Source: CAD feature listing. Evaluate the final solid. Frame: model axes, mm. A direction names the side the tool comes from. Give positions to 0.01 mm unless a question says otherwise; leave off trailing zeros. Write each loop counter-clockwise with the first axis right and the second up, starting at its lowest first coordinate (ties: lowest second). Pieces come first, ordered by that corner, then holes. Notation, with made-up numbers: (57, 35.5) -> (93, 35.5) arc R20 ccw to (93, 42.5) -> close; hole circle Ø1 at (24.25, 51.5). An arc over 180 degrees is marked (long way). Answer as a JSON object with one key per item and string values. Group by question number.
Item 1: Section query D-D on z = 3.75. Return the cut outline in (x, y), plus the area to 3 significant figures.
Item 2: Section query B-B on z = 18.25. Return the cut outline in (x, y), plus the area to 3 significant figures.
Item 3: Access query for faces 1 (the face through (8, 0, 2)), 2 (the face through (1.568, -4.748, 3.774)), 3 (the face through (7.654, -3.143, 7.395)), 4 (the face through (2.285, 3.584, 17.712)). Directions: +Z, -Z, +X, -X, +Y, -Y. A direction counts if a zero-diameter tool reaches every point of the face in a straight line with its end or side. Return the directions, or none.
Item 4: Pull-direction query (Y, two-part tool) for faces 5 (the face through (10.492, 3.304, 3.451)), 6 (the face through (-4, -3, 4)), 7 (the face through (-3, -2, 0)), 8 (the face through (-6.73, 4.42, 2.04)); classes: pulls with the +Y half, pulls with the -Y half, needs draft (parallel to the pull), parting line crosses it, or undercut.
Item 5: Section query C-C on x = -1.5. Return the cut outline in (y, z).
Item 6: First-contact query: pin 1 Ø3 at (y, z) = (-6, 5.5) entering from -X; pin 2 Ø6 at (y, z) = (2, 14) entering from -X; pin 3 Ø4 at (y, z) = (0, 4.5) entering from +X; pin 4 Ø1.5 at (x, z) = (-4.5, 18.5) entering from -Y. Flat tips, straight axial feed; report the tip coordinate or a pass-through.
Item 7: Ray query, probe 1 along X at (y, z) = (-3, 7.5); probe 2 along Y at (x, z) = (0, 6.25); probe 3 along Y at (x, z) = (0, 10.75). Return the intervals inside material, ascending. Write a range as from..to.
Item 8: Section query A-A on y = 0. Return the cut outline in (x, z).
from build123d import *

# Parameters (mm, degrees)
F0_R      = 11
F1_DEPTH  = 7
F2_R      = 9.5
F3_DEPTH  = 8
F4_R      = 4.25
F5_DEPTH  = 5.5
F6_R      = 3.25
F7_DEPTH  = 20.501
F10_R     = 1.75
F19_DEPTH = 6
F12_R     = 1.75
F20_DEPTH = 6
F14_R     = 1.75
F21_DEPTH = 6
F16_R     = 1.75
F22_DEPTH = 6
F18_R     = 1.75
F23_DEPTH = 6
F24_R     = 2
F25_DEPTH = 25


with BuildPart() as f1:
    # F0 (on Top) → F1 (new body)
    with BuildSketch(Plane.XY):
        Circle(F0_R)
    extrude(amount=F1_DEPTH)

    # F2 (on face) → F3 (join)
    with BuildSketch(Plane.XY.offset(7)):
        Circle(F2_R)
    extrude(amount=F3_DEPTH)

    # F4 (on face) → F5 (join)
    with BuildSketch(Plane.XY.offset(15)):
        Circle(F4_R)
    extrude(amount=F5_DEPTH)

    # F6 (on face) → F7 (cut, through all)
    with BuildSketch(Plane.XY.offset(20.5)):
        Circle(F6_R)
    extrude(amount=-F7_DEPTH, mode=Mode.SUBTRACT)

    # F10 (on line) → F19 (cut)
    with BuildSketch(Plane.YZ.offset(11)):
        with Locations((0, 3.75)):
            Circle(F10_R)
    extrude(amount=-F19_DEPTH, mode=Mode.SUBTRACT)

    # F12 (on line) → F20 (cut)
    with BuildSketch(Plane(origin=(3.3991869381, -10.4616216792, 0), x_dir=(-0.9510565163, -0.3090169944, 0), z_dir=(-0.3090169944, 0.9510565163, 0))):
        with Locations((0, 3.75)):
            Circle(F12_R)
    extrude(amount=F20_DEPTH, mode=Mode.SUBTRACT)

    # F14 (on face) → F21 (cut)
    with BuildSketch(Plane(origin=(-8.8991869381, -6.4656377752, 0), x_dir=(-0.5877852523, 0.8090169944, 0), z_dir=(0.8090169944, 0.5877852523, 0))):
        with Locations((0, 3.75)):
            Circle(F14_R)
    extrude(amount=F21_DEPTH, mode=Mode.SUBTRACT)

    # F16 (on face) → F22 (cut)
    with BuildSketch(Plane(origin=(-8.8991869381, 6.4656377752, 0), x_dir=(0.5877852523, 0.8090169944, 0), z_dir=(0.8090169944, -0.5877852523, 0))):
        with Locations((0, 3.75)):
            Circle(F16_R)
    extrude(amount=F22_DEPTH, mode=Mode.SUBTRACT)

    # F18 (on line) → F23 (cut)
    with BuildSketch(Plane(origin=(3.3991869381, 10.4616216792, 0), x_dir=(-0.9510565163, 0.3090169944, 0), z_dir=(0.3090169944, 0.9510565163, 0))):
        with Locations((0, 3.75)):
            Circle(F18_R)
    extrude(amount=-F23_DEPTH, mode=Mode.SUBTRACT)

    # F24 (on face) → F25 (cut)
    with BuildSketch(Plane(origin=(0, 0, 0), x_dir=(1, 0, 0), z_dir=(0, 0, -1))):
        with Locations((5.8068181818, 3.9090743921)):
            Circle(F24_R)
    extrude(amount=-F25_DEPTH, mode=Mode.SUBTRACT)


solid = f1.part
Worked answers:
{
 "1": {"outline": "(-9.81, -4.97) -> (-5.07, -1.52) -> (-3.02, -4.35) -> (-7.76, -7.8) arc R11 ccw to (1.69, -10.87) -> (-0.12, -5.3) -> (3.21, -4.21) -> (5.02, -9.79) arc R11 ccw to (10.86, -1.75) -> (5, -1.75) -> (5, 1.75) -> (10.86, 1.75) arc R11 ccw to (5.02, 9.79) -> (3.21, 4.21) -> (-0.12, 5.3) -> (1.69, 10.87) arc R11 ccw to (-7.76, 7.8) -> (-3.02, 4.35) -> (-5.07, 1.52) -> (-9.81, 4.97) arc R11 ccw to start; hole circle Ø6.5 at (0, 0); hole circle Ø4 at (5.81, -3.91)", "area": "230 mm^2"},
 "2": {"outline": "circle Ø8.5 at (0, 0); hole circle Ø6.5 at (0, 0)", "area": "23.6 mm^2"},
 "3": {"face 1": "+X", "face 2": "none", "face 3": "+Z, -Z", "face 4": "+Z"},
 "4": {"face 5": "parting line crosses it", "face 6": "undercut", "face 7": "needs draft", "face 8": "undercut"},
 "5": {"outline": "(-10.9, 0) -> (-2.88, 0) -> (-2.88, 20.5) -> (-3.98, 20.5) -> (-3.98, 15) -> (-9.38, 15) -> (-9.38, 7) -> (-10.9, 7) -> close; (2.88, 0) -> (10.9, 0) -> (10.9, 7) -> (9.38, 7) -> (9.38, 15) -> (3.98, 15) -> (3.98, 20.5) -> (2.88, 20.5) -> close"},
 "6": {"pin 1": "x = -10.04", "pin 2": "x = -9.5", "pin 3": "x = 11", "pin 4": "y = -2"},
 "7": {"probe 1": "-9.01..-1.25, 1.25..4.03, 7.59..9.01", "probe 2": "-11..-3.25, 3.25..11", "probe 3": "-9.5..-3.25, 3.25..9.5"},
 "8": {"outline": "(-11, 0) -> (-3.25, 0) -> (-3.25, 20.5) -> (-4.25, 20.5) -> (-4.25, 15) -> (-9.5, 15) -> (-9.5, 7) -> (-11, 7) -> close; (3.25, 0) -> (11, 0) -> (11, 2) -> (5, 2) -> (5, 5.5) -> (11, 5.5) -> (11, 7) -> (9.5, 7) -> (9.5, 15) -> (4.25, 15) -> (4.25, 20.5) -> (3.25, 20.5) -> close"}
}
